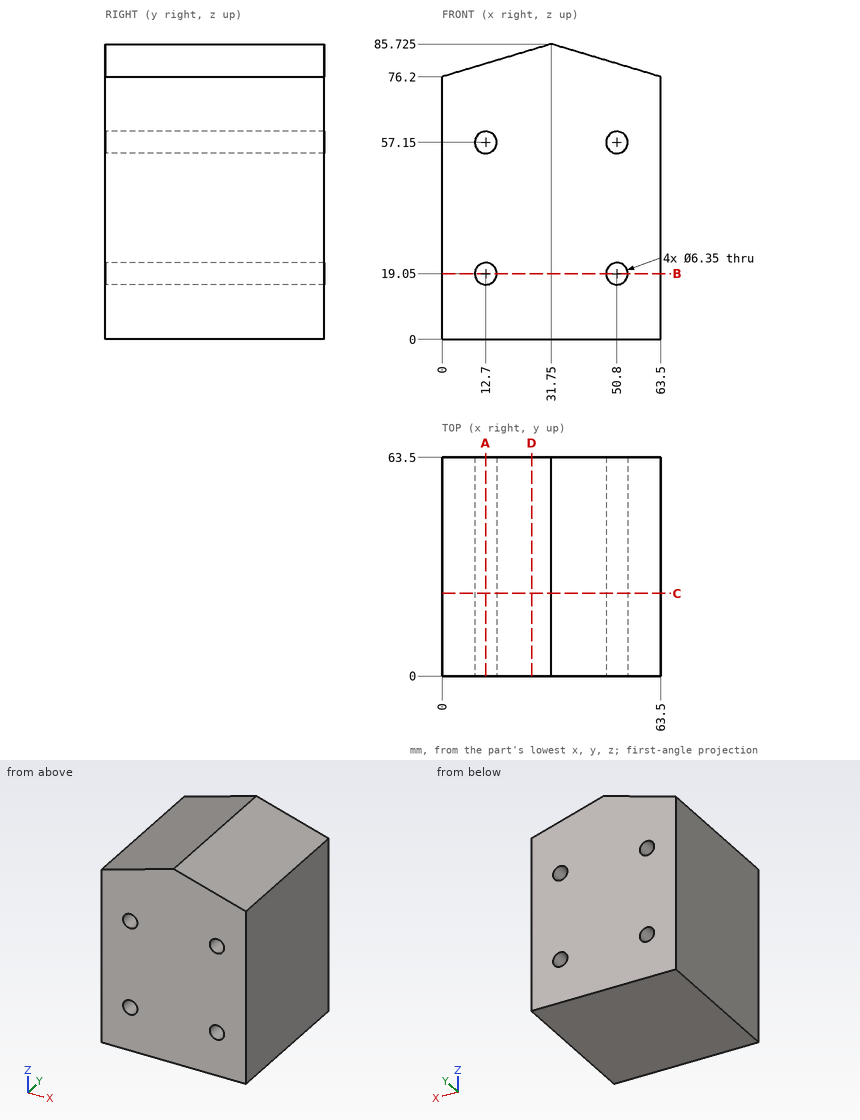
Answer from the drawing. Dimensions are ordinates in mm from the lowest x, y and z of the part. Coordinates: 2 decimals unless noted, no trailing zeros. Order: outer loops, then holes, each group sorted by start corner. A loop starts at its lowest first (then second) coordinate and runs counter-clockwise, first axis right, second up. Notation, with made-up numbers: (-17, 1.5) - (19, 1.5) arc R37 ccw to (19, 40.5) - close; hole circle Ø10 at (59.25, -8.75). An arc over 180 degrees is marked (long way). Put each result on its own line as item: value. Start each with the question number.
1) Find section B-B (z = 19.05). Give the vertices of the cut face in (x, y) (3 decimals).
2) Find section C-C (y = 24). Give the vertices of the cut face in (x, z) (3 decimals).
3) Find section A-A (x = 12.7). Give the vertices of the cut face in (y, z) (3 decimals).
4) Find the intervals of material crossed by line 1 (X direction, y = 38, z = 19); line 2 (Z direction, x = 12, y = 17); line 3 (Z direction, x = 50, y = 23), in increasing order. Write a range as from..to.
5) Find section D-D (x = 26). Give the vertices of the cut face in (y, z), plus the area to 3 significant figures.
6) A flat-ended cylindrical pin translates along its axis: pin 1 (10 mm diameter, centred on x = 12.7, z = 19.05, fed in from +Y). Find the tip coordinate at first contact, or state that the pin passes through.
Results list:
1. outline: (0, 0) - (9.525, 0) - (9.525, 63.5) - (0, 63.5) - close; (15.875, 0) - (47.625, 0) - (47.625, 63.5) - (15.875, 63.5) - close; (53.975, 0) - (63.5, 0) - (63.5, 63.5) - (53.975, 63.5) - close
2. outline: (0, 0) - (63.5, 0) - (63.5, 76.2) - (31.75, 85.725) - (0, 76.2) - close; hole circle Ø6.35 at (12.7, 19.05); hole circle Ø6.35 at (12.7, 57.15); hole circle Ø6.35 at (50.8, 19.05); hole circle Ø6.35 at (50.8, 57.15)
3. outline: (0, 0) - (63.5, 0) - (63.5, 15.875) - (0, 15.875) - close; (0, 22.225) - (63.5, 22.225) - (63.5, 53.975) - (0, 53.975) - close; (0, 60.325) - (63.5, 60.325) - (63.5, 80.01) - (0, 80.01) - close
4. line 1: x = 0..9.53, 15.87..47.63, 53.97..63.5
4. line 2: z = 0..15.95, 22.15..54.05, 60.25..79.8
4. line 3: z = 0..15.98, 22.12..54.08, 60.22..80.25
5. outline: (0, 0) - (63.5, 0) - (63.5, 84) - (0, 84) - close
5. area: 5,330 mm^2
6. pin 1: stops at y = 63.5
